```python
from build123d import *

# Parameters (mm, degrees)
F0_R     = 2.5
F1_DEPTH = 3.5
F2_R     = 2.5
F3_DEPTH = 6.5


with BuildPart() as f1:
    # F0 (on Front) → F1 (new body, symmetric)
    with BuildSketch(Plane.XZ):
        with BuildLine():
            ThreePointArc((54.518331, 30.600595), (55.434331, 22.08937), (54.518331, 13.578145))
            ThreePointArc((54.518331, 13.578145), (61.358031, 5.088681), (68.197731, 13.578145))
            ThreePointArc((68.197731, 13.578145), (67.281731, 22.08937), (68.197731, 30.600595))
            ThreePointArc((68.197731, 30.600595), (61.358031, 39.090059), (54.518331, 30.600595))
        make_face()
        with Locations((61.358031, 12.088681)):
            Circle(F0_R, mode=Mode.SUBTRACT)
        with Locations((61.358031, 32.090059)):
            Circle(F0_R, mode=Mode.SUBTRACT)
    extrude(amount=F1_DEPTH, both=True)

    # F2 (on Front) → F3 (join, symmetric)
    with BuildSketch(Plane.XZ):
        with Locations((61.358031, 32.090059)):
            Circle(F2_R)
        with Locations((61.358031, 12.088681)):
            Circle(F2_R)
    extrude(amount=F3_DEPTH, both=True)


solid = f1.part
```
Work out the finished part from the listing and answer in its coordinate system (mm). A direction names the side the tool comes from. Coordinates: 2 decimals unless noted, no trailing zeros. Loops run counter-clockwise (first coordinate to the right, second up) from the corner with the lowest first, then second, coordinate; pieces in that order, holes last.
1) Flat-ended cylindrical pins translate along their axes: pin 1 (4 mm diameter, centred on x = 57, y = 3, fed in from -Z); pin 2 (1.5 mm diameter, centred on y = 3, z = 26, fed in from +X); pin 3 (6 mm diameter, centred on y = -4, z = 29, fed in from +X). Find the tip coordinate at first contact, or state that the pin passes through.
Results:
pin 1: stops at z = 5.5
pin 2: stops at x = 67.55
pin 3: stops at x = 68.36
2) Section C-C (y = 1.5) is taken. Give the vertices of the cut face in (x, z).
Results:
outline: (54.52, 13.58) arc R7 ccw (long way) to (68.2, 13.58) arc R40 cw to (68.2, 30.6) arc R7 ccw (long way) to (54.52, 30.6) arc R40 cw to start
3) For faces 1 (the cylindrical face through (59.515, -4.979, 33.78)), 2 (the cylindrical face through (55.434, -0.049, 22.209)), 3 (the cylindrical face through (58.86, 4.98, 12.2)), determine the directions among +Z, -Z, +X, -X, +Y, -Y from which every point of the face is accessible in a straight line to the end or side of a thin tool.
Results:
face 1: -Y
face 2: -X, +Y, -Y
face 3: +Y
4) Section A-A (y = -5) is taken. Give the vertices of the cut face in (x, z).
Results:
outline: circle Ø5 at (61.36, 12.09); circle Ø5 at (61.36, 32.09)
5) Section D-D (z = 15.5) is taken. Give the vertices of the cut face in (x, y).
Results:
outline: (54.89, -3.5) - (67.83, -3.5) - (67.83, 3.5) - (54.89, 3.5) - close
6) Consider probe 1 along Y at (x, z) = (58, 25); probe 2 along Z at (x, y) = (62.75, 6.25); probe 3 along Z at (x, y) = (58.25, 3). Determine where each line is inside the solid, lowest interval first.
Results:
probe 1: y = -3.5 to 3.5
probe 2: z = 10.01 to 14.17, 30.01 to 34.17
probe 3: z = 5.82 to 38.36
7) Section B-B (x = 61.75) is taken. Give the vertices of the cut face in (y, z).
Results:
outline: (-6.5, 9.62) - (-3.5, 9.62) - (-3.5, 5.1) - (3.5, 5.1) - (3.5, 9.62) - (6.5, 9.62) - (6.5, 14.56) - (3.5, 14.56) - (3.5, 29.62) - (6.5, 29.62) - (6.5, 34.56) - (3.5, 34.56) - (3.5, 39.08) - (-3.5, 39.08) - (-3.5, 34.56) - (-6.5, 34.56) - (-6.5, 29.62) - (-3.5, 29.62) - (-3.5, 14.56) - (-6.5, 14.56) - close
